The drawing under review shows one solid part. Ordinate dimensions are in mm from its lowest x, y, z. A direction names the side the tool comes from. Coordinates: 2 decimals unless noted, no trailing zeros. Write each loop counter-clockwise with the first axis right and the second up, starting at its lowest first coordinate (ties: lowest second). Pieces come first, ordered by that corner, then holes.
Q1. Add section B-B, the plane y = 5.08. Give the number of separate pieces and of enclosed holes in the cut face, plus the area to 3 significant figures.
Q2. Add section C-C, the plane x = 34. Give the boundary of the cut face in (y, z).
Q3. Add section A-A, the plane z = 31.75. Give the boundary of the cut face in (x, y), plus the area to 3 significant figures.
Q4. Clearance check with flat-ended pins moving along their axes: pin 1 Ø5.5 at (x, y) = (58.42, 5.08) entering from -Z; pin 2 Ø3 at (y, z) = (6.5, 7.5) entering from +X; pin 3 Ø5 at (x, y) = (11, 7) entering from -Z. State where each tip first meets the part, or that it passes through.
Q5. Add section D-D, the plane x = 5.08. Give the boundary of the cut face in (y, z), plus the area to 3 significant figures.
Q6. To check wall thickness, follow probe 1 along Y at (x, z) = (5, 31); probe 2 along X at (y, z) = (7.5, 35.5); probe 3 along X at (y, z) = (1.5, 4). State the ranges of each line that lie inside material, in increasing order.
Q7. Machinability: for the marked faces 4, 5 and 6, which of the approach directions +Z, -Z, +X, -X, +Y, -Y give a long, thin tool a straight path to every point of the face, cutting with its end or side? Answer none if there is none.
Q8. The part is to be moulded in two halves that separate along Y. For the marked faces 1, 2 and 3, say which applies: +Y half, -Y half, draft (parallel to the pull), parting line (faces both ways), or undercut.
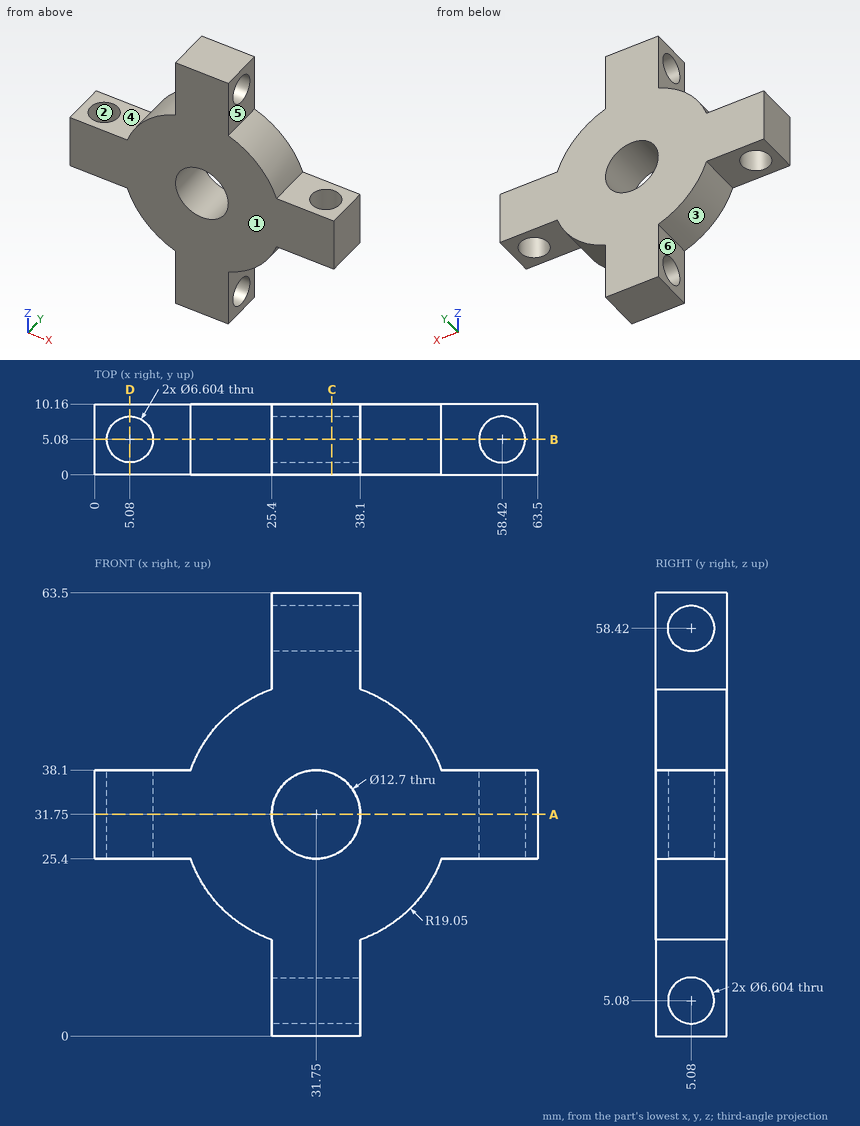
Here are the results:
1. separate pieces: 5
1. enclosed holes: 1
1. area: 1,340 mm2
2. outline: (0, 0) - (10.16, 0) - (10.16, 25.81) - (0, 25.81) - close; (0, 37.69) - (10.16, 37.69) - (10.16, 63.5) - (0, 63.5) - close; hole circle Ø6.6 at (5.08, 5.08); hole circle Ø6.6 at (5.08, 58.42)
3. outline: (0, 0) - (25.4, 0) - (25.4, 10.16) - (0, 10.16) - close; (38.1, 0) - (63.5, 0) - (63.5, 10.16) - (38.1, 10.16) - close; hole circle Ø6.6 at (5.08, 5.08); hole circle Ø6.6 at (58.42, 5.08)
3. area: 448 mm2
4. pin 1: passes through
4. pin 2: stops at x = 38.1
4. pin 3: stops at z = 25.4
5. outline: (0, 25.4) - (1.78, 25.4) - (1.78, 38.1) - (0, 38.1) - close; (8.38, 25.4) - (10.16, 25.4) - (10.16, 38.1) - (8.38, 38.1) - close
5. area: 45.2 mm2
6. probe 1: y = 0 to 1.78, 8.38 to 10.16
6. probe 2: x = 0 to 2.83, 7.33 to 26.63, 36.87 to 56.17, 60.67 to 63.5
6. probe 3: x = 25.4 to 38.1
7. face 4: +Z, -X, +Y, -Y
7. face 5: +Z, +X, +Y, -Y
7. face 6: -Z, -X, +Y, -Y
8. face 1: -Y half
8. face 2: undercut
8. face 3: draft
